from build123d import *

# Parameters (mm, degrees)
F1_DEPTH = 25


with BuildPart() as f1:
    # F0 (on Top) → F1 (new body)
    with BuildSketch(Plane.XY):
        with BuildLine():
            Line((-28.602151, -27.943548), (-28.602151, -62.943548))
            Line((-28.602151, -62.943548), (1.397849, -62.943548))
            Line((1.397849, -62.943548), (1.397849, 57.056452))
            Line((1.397849, 57.056452), (-3.602151, 57.056452))
            ThreePointArc((-3.602151, 57.056452), (-7.137685, 55.591986), (-8.602151, 52.056452))
            Line((-8.602151, 52.056452), (-8.602151, 42.056452))
            Line((-8.602151, 42.056452), (-13.602151, 42.056452))
            ThreePointArc((-13.602151, 42.056452), (-17.137685, 40.591986), (-18.602151, 37.056452))
            Line((-18.602151, 37.056452), (-18.602151, 12.056452))
            ThreePointArc((-18.602151, 12.056452), (-22.137685, 10.591986), (-23.602151, 7.056452))
            Line((-23.602151, 7.056452), (-23.602151, -22.943548))
            ThreePointArc((-23.602151, -22.943548), (-27.137685, -24.408014), (-28.602151, -27.943548))
        make_face()
    extrude(amount=F1_DEPTH)


solid = f1.part
Here's how the part is built. I have some questions about the finished solid (model axes, mm). A direction names the side the tool comes from. Round coordinates to 2 decimals unless told otherwise and drop trailing zeros. Write each loop counter-clockwise with the first axis right and the second up, starting at its lowest first coordinate (ties: lowest second). Pieces come first, ordered by that corner, then holes.
1. For faces 1 (the flat face through (1.398, -4, 12)), 2 (the flat face through (-8.602, 47, 12)), which set-ups out of +Z, -Z, +X, -X, +Y, -Y let a thin tool reach every point of the face, with its end or its side?
2. Will these pins go through, and if not, where does the flat tip stop? pin 1 Ø7.5 at (y, z) = (-2.5, 15.5) entering from -X; pin 2 Ø4 at (x, z) = (-11, 10) entering from +Y; pin 3 Ø3 at (y, z) = (48, 8) entering from -X.
3. Suppose I cut it at C-C (x = -26). List the corners of the cut face in (y, z) for me, and give its area (3 significant figures).
4. I need wall thicknesses on L1, parallel to X at y = 44, z = 15.75; L2, parallel to X at y = 15, z = 20.5; L3, parallel to Y at x = -11, z = 13.75. Which ranges of each line are inside material? Lowest first, please.
5. Suppose I cut it at A-A (z = 16.25). List the corners of the cut face in (x, y) for me, and give its area (3 significant figures).
6. Suppose I cut it at B-B (y = 21). List the corners of the cut face in (x, z) for me.
Answer sheet:
1. face 1: +Z, -Z, +X, +Y, -Y
1. face 2: +Z, -Z, -X, +Y
2. pin 1: stops at x = -23.6
2. pin 2: stops at y = 42.06
2. pin 3: stops at x = -8.6
3. outline: (-62.94, 0) - (-23.56, 0) - (-23.56, 25) - (-62.94, 25) - close
3. area: 985 mm2
4. L1: x = -8.6 to 1.4
4. L2: x = -18.6 to 1.4
4. L3: y = -62.94 to 42.06
5. outline: (-28.6, -62.94) - (1.4, -62.94) - (1.4, 57.06) - (-3.6, 57.06) arc R5 ccw to (-8.6, 52.06) - (-8.6, 42.06) - (-13.6, 42.06) arc R5 ccw to (-18.6, 37.06) - (-18.6, 12.06) arc R5 ccw to (-23.6, 7.06) - (-23.6, -22.94) arc R5 ccw to (-28.6, -27.94) - close
5. area: 2,800 mm2
6. outline: (-18.6, 0) - (1.4, 0) - (1.4, 25) - (-18.6, 25) - close
